Source: three-view drawing plus pictorial views. Frame: mm from the lowest corner of the part. Give positions to 0.01 mm unless a question says otherwise; leave off trailing zeros. Order: outer loops, then holes, each group sorted by start corner. A loop starts at its lowest first (then second) coordinate and runs counter-clockwise, first axis right, second up. Notation, with made-up numbers: (-10, 37.25) -> (9, 37.25) arc R15 ccw to (9, 60.25) -> close; hole circle Ø6 at (85, 6). An arc over 180 degrees is marked (long way). One line per question, with ' | ' between items.
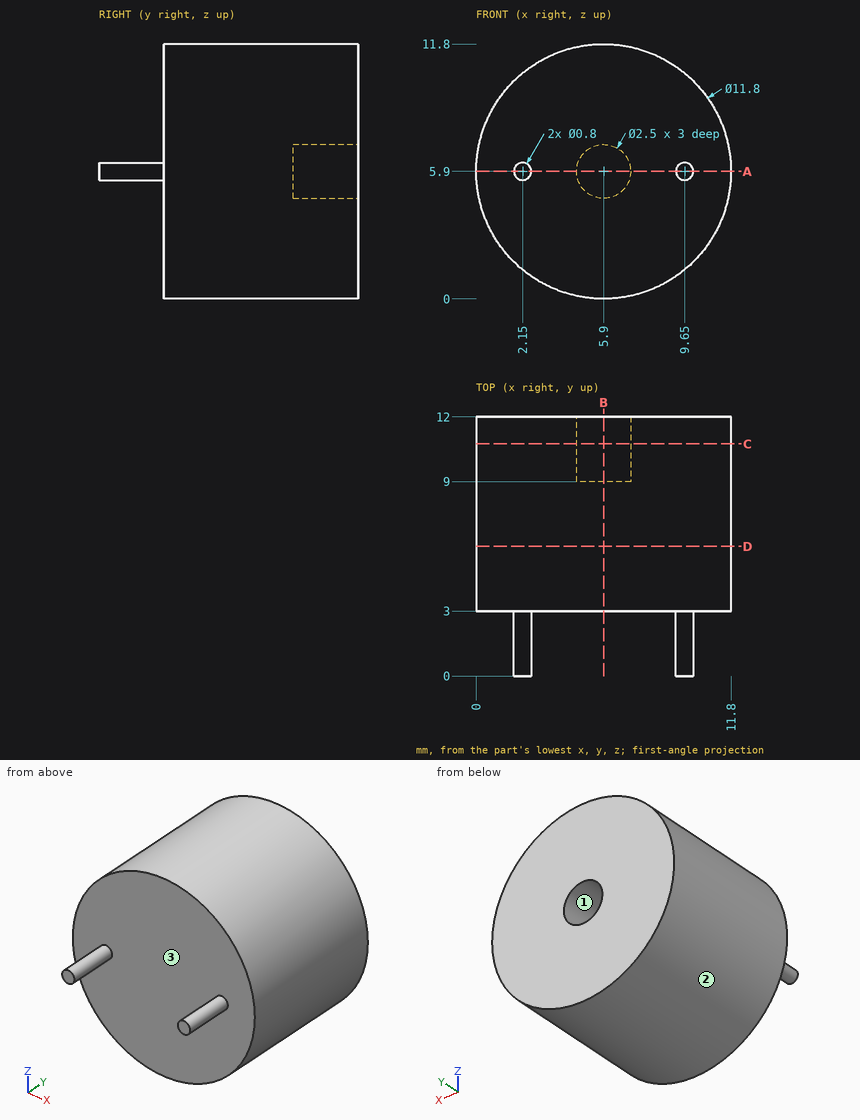
1) Pull-direction query (Z, two-part tool) for the marked faces 1, 2 and 3; classes: +Z half, -Z half, draft (parallel to the pull), parting line (faces both ways), or undercut.
Check result:
face 1: undercut | face 2: parting line | face 3: draft
2) Material intervals for probe 1 along Z at (x, y) = (5.9, 10.4); probe 2 along Y at (x, z) = (7.5, 10.25), sorted ascending. Write a range as from..to.
Check result:
probe 1: z = 0..4.65, 7.15..11.8 | probe 2: y = 3..12
3) Section C-C on y = 10.75. Return loops of the section in (x, z), plus the area to 3 significant figures.
Check result:
outline: circle Ø11.8 at (5.9, 5.9); hole circle Ø2.5 at (5.9, 5.9) | area: 104 mm^2
4) Section A-A on z = 5.9. Return loops of the section in (x, y), plus the area to 4 significant figures.
Check result:
outline: (0, 3) -> (1.75, 3) -> (1.75, 0) -> (2.55, 0) -> (2.55, 3) -> (9.25, 3) -> (9.25, 0) -> (10.05, 0) -> (10.05, 3) -> (11.8, 3) -> (11.8, 12) -> (7.15, 12) -> (7.15, 9) -> (4.65, 9) -> (4.65, 12) -> (0, 12) -> close | area: 103.5 mm^2
5) Section D-D on y = 6. Return loops of the section in (x, z).
Check result:
outline: circle Ø11.8 at (5.9, 5.9)
6) Section B-B on x = 5.9. Return loops of the section in (y, z), plus the area to 3 significant figures.
Check result:
outline: (3, 0) -> (12, 0) -> (12, 4.65) -> (9, 4.65) -> (9, 7.15) -> (12, 7.15) -> (12, 11.8) -> (3, 11.8) -> close | area: 98.7 mm^2
7) Contact query for flat-ended pins moving along their axis: pin 1 Ø3.5 at (x, z) = (8, 7.5) entering from -Y; pin 2 Ø6 at (y, z) = (9, 10) entering from +X; pin 3 Ø5 at (x, y) = (10, 4) entering from -Z. Output: stop coordinate, or through.
Check result:
pin 1: stops at y = 3 | pin 2: stops at x = 11.7 | pin 3: stops at z = 0.22
